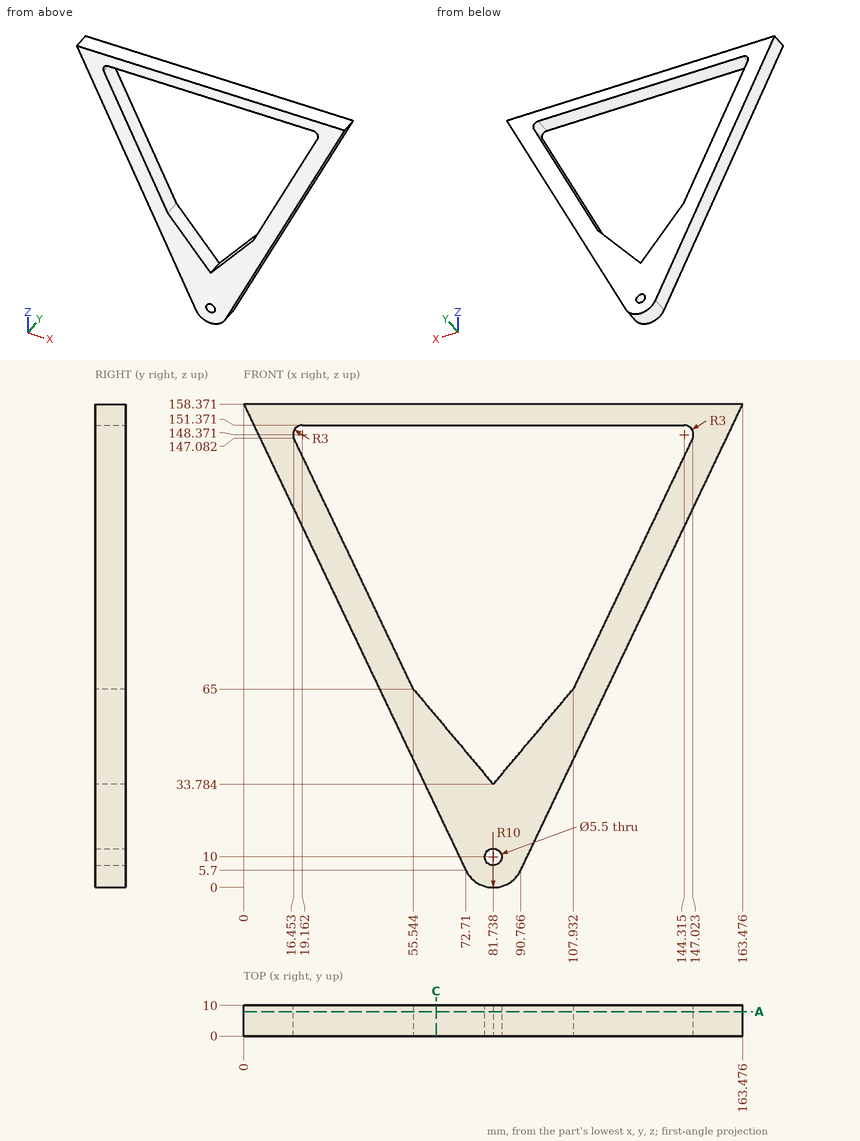
For this review, use the dimensioned drawing (mm, ordinates from the lowest corner) and the shaded views. Coordinates: 2 decimals unless noted, no trailing zeros. Write each loop counter-clockwise with the first axis right and the second up, starting at its lowest first coordinate (ties: lowest second). Pieces come first, ordered by that corner, then holes. Notation, with made-up numbers: (-13, -9) - (27, -9) arc R9 ccw to (27, 2) - close; hole circle Ø7 at (72, 73.5). An arc over 180 degrees is marked (long way). Answer as a JSON object with one key per item and string values. Group by question number.
1. Clearance check with flat-ended pins moving along their axes: pin 1 Ø5 at (x, y) = (60.5, 3) entering from -Z (1 decimal); pin 2 Ø10 at (x, z) = (51.5, 78.5) entering from +Y; pin 3 Ø2 at (x, y) = (121.5, 6.5) entering from -Z (1 decimal). State where each tip first meets the part, or that it passes through.
2. To check wall thickness, follow probe 1 along X at (y, z) = (7.25, 57) (1 decimal); probe 2 along Z at (x, y) = (21, 1.5) (1 decimal); probe 3 along Z at (x, y) = (74, 2.75) (1 decimal). State the ranges of each line that lie inside material, in increasing order.
3. Add section A-A (y = 8). Give the number of separate pieces and of enclosed holes in the cut face, plus the area to 3 significant figures.
4. Add section C-C (x = 63). Give the boundary of the cut face in (y, z) (1 decimal).
Findings:
{
 "1": {"pin 1": "z = 26.1", "pin 2": "y = 10", "pin 3": "z = 68.1"},
 "2": {"probe 1": "48.3 to 62.3, 101.2 to 115.2", "probe 2": "114.3 to 137.5, 151.4 to 158.4", "probe 3": "3.7 to 43, 151.4 to 158.4"},
 "3": {"separate pieces": "1", "enclosed holes": "2", "area": "5,020 mm²"},
 "4": {"outline": "(0, 26.1) - (10, 26.1) - (10, 56.1) - (0, 56.1) - close; (0, 151.4) - (10, 151.4) - (10, 158.4) - (0, 158.4) - close"}
}
